The model under review builds one solid part; all positions refer to its coordinate system, in mm. Coordinates: 2 decimals unless noted, no trailing zeros. Write each loop counter-clockwise with the first axis right and the second up, starting at its lowest first coordinate (ties: lowest second). Pieces come first, ordered by that corner, then holes. Notation, with made-up numbers: M -32,80 L 14,80 A3 ccw 14,84 Z; hole C 0,0 d1. An arc over 180 degrees is marked long. Answer as a JSON object with one key per item and string values.
```python
from build123d import *

# Parameters (mm, degrees)
F0_R     = 1.7272
F1_DEPTH = 12.7
F2_R     = 1.7272
F3_DEPTH = 12.7
F4_R     = 6.35


with BuildPart() as f1:
    # F0 (on Top) → F1 (new body)
    with BuildSketch(Plane.XY):
        Polygon((-177.8, 431.8), (-177.8, -431.8), (-381, -431.8), (-381, -1193.8), (381, -1193.8), (381, -431.8), (177.8, -431.8), (177.8, 431.8), (381, 431.8), (381, 1193.8), (-381, 1193.8), (-381, 431.8), align=None)
        with Locations((-249.2375, -1062.0375)):
            Circle(F0_R, mode=Mode.SUBTRACT)
        with Locations((-193.675, -819.15)):
            Circle(F0_R, mode=Mode.SUBTRACT)
        with Locations((-138.1125, -1062.0375)):
            Circle(F0_R, mode=Mode.SUBTRACT)
        with Locations((-249.2375, -576.2625)):
            Circle(F0_R, mode=Mode.SUBTRACT)
        with Locations((-138.1125, -576.2625)):
            Circle(F0_R, mode=Mode.SUBTRACT)
        with Locations((-46.0375, -300.0375)):
            Circle(F0_R, mode=Mode.SUBTRACT)
        with Locations((138.1125, -1062.0375)):
            Circle(F0_R, mode=Mode.SUBTRACT)
        with Locations((249.2375, -1062.0375)):
            Circle(F0_R, mode=Mode.SUBTRACT)
        with Locations((193.675, -819.15)):
            Circle(F0_R, mode=Mode.SUBTRACT)
        with Locations((46.0375, -300.0375)):
            Circle(F0_R, mode=Mode.SUBTRACT)
        with Locations((138.1125, -576.2625)):
            Circle(F0_R, mode=Mode.SUBTRACT)
        with Locations((249.2375, -576.2625)):
            Circle(F0_R, mode=Mode.SUBTRACT)
        with Locations((-249.2375, 576.2625)):
            Circle(F0_R, mode=Mode.SUBTRACT)
        with Locations((-46.0375, 0)):
            Circle(F0_R, mode=Mode.SUBTRACT)
        with Locations((-138.1125, 576.2625)):
            Circle(F0_R, mode=Mode.SUBTRACT)
        with Locations((-46.0375, 300.0375)):
            Circle(F0_R, mode=Mode.SUBTRACT)
        with Locations((-193.675, 819.15)):
            Circle(F0_R, mode=Mode.SUBTRACT)
        with Locations((-249.2375, 1062.0375)):
            Circle(F0_R, mode=Mode.SUBTRACT)
        with Locations((-138.1125, 1062.0375)):
            Circle(F0_R, mode=Mode.SUBTRACT)
        with Locations((46.0375, 0)):
            Circle(F0_R, mode=Mode.SUBTRACT)
        with Locations((46.0375, 300.0375)):
            Circle(F0_R, mode=Mode.SUBTRACT)
        with Locations((138.1125, 576.2625)):
            Circle(F0_R, mode=Mode.SUBTRACT)
        with Locations((249.2375, 576.2625)):
            Circle(F0_R, mode=Mode.SUBTRACT)
        with Locations((138.1125, 1062.0375)):
            Circle(F0_R, mode=Mode.SUBTRACT)
        with Locations((193.675, 819.15)):
            Circle(F0_R, mode=Mode.SUBTRACT)
        with Locations((249.2375, 1062.0375)):
            Circle(F0_R, mode=Mode.SUBTRACT)
    extrude(amount=F1_DEPTH)

    # F2 (on face) → F3 (cut, through all)
    with BuildSketch(Plane.XY.offset(12.7)):
        with Locations((0, -438.15)):
            Circle(F2_R)
        with Locations((-374.65, -438.15)):
            Circle(F2_R)
        with Locations((374.65, -438.15)):
            Circle(F2_R)
        with Locations((0, -1187.45)):
            Circle(F2_R)
        with Locations((0, -812.8)):
            Circle(F2_R)
        with Locations((374.65, 438.15)):
            Circle(F2_R)
        with Locations((0, 438.15)):
            Circle(F2_R)
        with Locations((0, 812.8)):
            Circle(F2_R)
        with Locations((0, 1187.45)):
            Circle(F2_R)
        with Locations((-374.65, 438.15)):
            Circle(F2_R)
        with Locations((-10.31875, 374.65)):
            Circle(F2_R)
        with Locations((-10.31875, 342.9)):
            Circle(F2_R)
        with Locations((10.31875, 342.9)):
            Circle(F2_R)
        with Locations((10.31875, 374.65)):
            Circle(F2_R)
        with Locations((-10.31875, -336.55)):
            Circle(F2_R)
        with Locations((10.31875, -336.55)):
            Circle(F2_R)
        with Locations((10.31875, -368.3)):
            Circle(F2_R)
        with Locations((-10.31875, -368.3)):
            Circle(F2_R)
    extrude(amount=-F3_DEPTH, mode=Mode.SUBTRACT)

    # F4
    f4_edges = [f1.edges().sort_by_distance(p)[0] for p in [
        (-381, -431.8, 6.35),
        (381, -431.8, 6.35),
        (381, -1193.8, 6.35),
        (-381, -1193.8, 6.35),
        (-381, 431.8, 6.35),
        (381, 431.8, 6.35),
        (381, 1193.8, 6.35),
        (-381, 1193.8, 6.35),
    ]]
    fillet(f4_edges, radius=F4_R)


solid = f1.part
```
(1) Wall thickness on line 1 along X through (y, z) = (-438.15, 8); line 2 along Y through (x, z) = (374.65, 6.5); line 3 along Y through (x, z) = (-216, 1): over which ranges is each line inside the solid? List them lowest first. Write a range as from..to.
Results list:
{"line 1": "-381..-376.38, -372.92..-1.73, 1.73..372.92, 376.38..381", "line 2": "-1193.8..-439.88, -436.42..-431.8, 431.8..436.42, 439.88..1193.8", "line 3": "-1193.8..-431.8, 431.8..1193.8"}
(2) Add section B-B on y = 275. Give the boundary of the cut face in (x, z).
Results list:
{"outline": "M -177.8,0 L 177.8,0 L 177.8,12.7 L -177.8,12.7 Z"}
(3) For pin 1 Ø6 at (y, z) = (424.5, 9) entering from +X; pin 2 Ø2 at (y, z) = (435.5, 3.5) entering from -X, all flat-tipped, find the tip position at first contact; note any pin that passes through.
Results list:
{"pin 1": "x = 177.8", "pin 2": "x = -380.78"}
(4) Add section C-C on z = 3.5. Count the separate pieces of the cut face and the enclosed holes in it, and give its area (3 significant figures).
Results list:
{"separate pieces": "1", "enclosed holes": "44", "area": "1,470,000 mm²"}
(5) Add section A-A on x = -334. Give the boundary of the cut face in (y, z).
Results list:
{"outline": "M -1193.8,0 L -431.8,0 L -431.8,12.7 L -1193.8,12.7 Z; M 431.8,0 L 1193.8,0 L 1193.8,12.7 L 431.8,12.7 Z"}
